from build123d import *

# Parameters (mm, degrees)
SKETCH1_R           = 49
BOSS_EXTRUDE1_DEPTH = 24.5
SKETCH2_R           = 24
BOSS_EXTRUDE2_DEPTH = 1.7
SKETCH3_R           = 18.5
BOSS_EXTRUDE3_DEPTH = 0.8
SKETCH4_R           = 35.5
BOSS_EXTRUDE4_DEPTH = 11
CIRPATTERN1_COUNT   = 8
CIRPATTERN2_COUNT   = 6
SKETCH20_R          = 1.5
CUT_EXTRUDE1_DEPTH  = 3.5
SKETCH21_R          = 2
BOSS_EXTRUDE5_DEPTH = 2.5
CIRPATTERN3_COUNT   = 3


with BuildPart() as part:
    # Sketch1 → Boss-Extrude1 (new body)
    with BuildSketch(Plane(origin=(0, 0, 0), x_dir=(1, 0, 0), z_dir=(0, 1, 0))):
        Circle(SKETCH1_R)
    extrude(amount=BOSS_EXTRUDE1_DEPTH)

    # Sketch2 → Boss-Extrude2 (add)
    with BuildSketch(Plane(origin=(0, 24.5, 0), x_dir=(1, 0, 0), z_dir=(0, 1, 0))):
        Circle(SKETCH2_R)
    extrude(amount=BOSS_EXTRUDE2_DEPTH)

    # Sketch3 → Boss-Extrude3 (add)
    with BuildSketch(Plane(origin=(0, 26.2, 0), x_dir=(1, 0, 0), z_dir=(0, 1, 0))):
        Circle(SKETCH3_R)
    extrude(amount=BOSS_EXTRUDE3_DEPTH)

    # Sketch4 → Boss-Extrude4 (add)
    with BuildSketch(Plane.XZ):
        Circle(SKETCH4_R)
    extrude(amount=BOSS_EXTRUDE4_DEPTH)

    # Sketch13 → 3.0mm Dowel Hole1 (revolve, cut)
    with BuildSketch(Plane(origin=(-39.264880132, 0, 16.264045876), x_dir=(0, 0, -1), z_dir=(1, 0, 0))):
        Polygon((0, 0), (0, 3.901290929), (1.5, 3), (1.5, 0), align=None)
    f_3_0mm_dowel_hole1 = revolve(axis=Axis((-39.264880132, -6.35, 16.264045876), (0, 1, 0)), mode=Mode.SUBTRACT)

    # CirPattern1: 3.0mm Dowel Hole1 ×8 about axis
    cirpattern1_axis = Axis((0, 0, 0), (0, 1, 0))
    for i in range(1, CIRPATTERN1_COUNT):
        add(f_3_0mm_dowel_hole1.rotate(cirpattern1_axis, i * 360 / CIRPATTERN1_COUNT), mode=Mode.SUBTRACT)

    # Sketch15 → 4.0mm Dowel Hole1 (revolve, cut)
    with BuildSketch(Plane(origin=(-15, 27, 0), x_dir=(0, 0, 1), z_dir=(1, 0, 0))):
        Polygon((0, 0), (0, 5.701721238), (2, 4.5), (2, 0), align=None)
    f_4_0mm_dowel_hole1 = revolve(axis=Axis((-15, 33.35, 0), (0, -1, 0)), mode=Mode.SUBTRACT)

    # CirPattern2: 4.0mm Dowel Hole1 ×6 about axis, 3 skipped
    cirpattern2_axis = Axis((0, -12.925, 0), (0, 1, 0))
    add([f_4_0mm_dowel_hole1.rotate(cirpattern2_axis, i * 360 / CIRPATTERN2_COUNT) for i in range(1, CIRPATTERN2_COUNT) if i not in (1, 3, 5)], mode=Mode.SUBTRACT)

    # Sketch20 → Cut-Extrude1 (cut)
    with BuildSketch(Plane(origin=(0, 24.5, 0), x_dir=(1, 0, 0), z_dir=(0, 1, 0))):
        with Locations((39.264880132, -16.264045876)):
            Circle(SKETCH20_R)
        with Locations((16.264045876, -39.264880132)):
            Circle(SKETCH20_R)
        with Locations((-16.264045876, -39.264880132)):
            Circle(SKETCH20_R)
        with Locations((-39.264880132, -16.264045876)):
            Circle(SKETCH20_R)
        with Locations((-39.264880132, 16.264045876)):
            Circle(SKETCH20_R)
        with Locations((-16.264045876, 39.264880132)):
            Circle(SKETCH20_R)
        with Locations((16.264045876, 39.264880132)):
            Circle(SKETCH20_R)
        with Locations((39.264880132, 16.264045876)):
            Circle(SKETCH20_R)
    extrude(amount=-CUT_EXTRUDE1_DEPTH, mode=Mode.SUBTRACT)

    # Sketch21 → Boss-Extrude5 (add)
    with BuildSketch(Plane(origin=(0, 27, 0), x_dir=(1, 0, 0), z_dir=(0, 1, 0))):
        with Locations((-7.125, 12.340862004)):
            Circle(SKETCH21_R)
    boss_extrude5 = extrude(amount=BOSS_EXTRUDE5_DEPTH)

    # CirPattern3: Boss-Extrude5 ×3 about axis
    cirpattern3_axis = Axis((0, 0, 0), (0, 1, 0))
    for i in range(1, CIRPATTERN3_COUNT):
        add(boss_extrude5.rotate(cirpattern3_axis, i * 360 / CIRPATTERN3_COUNT))


solid = part.part
Work out the finished part from the listing and answer in its coordinate system (mm). A direction names the side the tool comes from. Round coordinates to 2 decimals unless told otherwise and drop trailing zeros. Loops run counter-clockwise (first coordinate to the right, second up) from the corner with the lowest first, then second, coordinate; pieces in that order, holes last. Notation, with made-up numbers: (20.5, 66.5) - (40.5, 66.5) arc R21 cw to (40.5, 90.5) - close; hole circle Ø1 at (-32.75, 42.25). An arc over 180 degrees is marked (long way). One line per item, written item: value.
Q1. Find section A-A on x = 0. Give the vertices of the cut face in (y, z).
Check values:
outline: (-11, -35.5) - (0, -35.5) - (0, -49) - (24.5, -49) - (24.5, -24) - (26.2, -24) - (26.2, -18.5) - (27, -18.5) - (27, 18.5) - (26.2, 18.5) - (26.2, 24) - (24.5, 24) - (24.5, 49) - (0, 49) - (0, 35.5) - (-11, 35.5) - close
Q2. The mould has two halves that part along X. Classify faces 4 (the conical face through (-16.321, 3.745, -39.011)), 5 (the cylindrical face through (-7.696, -5.423, -34.656)), 6 (the flat face through (21, 24.5, -12)): +X half, -X half, draft (parallel to the pull), parting line (faces both ways), or undercut.
Check values:
face 4: undercut
face 5: parting line
face 6: draft
Q3. Find section D-D on z = 43. Give the vertices of the cut face in (x, y).
Check values:
outline: (-23.49, 0) - (23.49, 0) - (23.49, 24.5) - (-23.49, 24.5) - close
Q4. Each of these flat-tipped pins is pushed along its axis until it touches: pin 1 Ø1.5 at (x, z) = (-16, 40) entering from +Y; pin 2 Ø1.5 at (x, z) = (16.5, -39.5) entering from +Y; pin 3 Ø1.8 at (x, z) = (39.26, 16.26) entering from -Y. Where does it stop, or does it pass through?
Check values:
pin 1: y = 24.5
pin 2: y = 21
pin 3: y = 3.36
Q5. Straight lines are drawn through the part: probe 1 along Y at (x, z) = (25.5, 9); probe 2 along X at (y, z) = (23, 0); probe 3 along Y at (x, z) = (11, 42). For each, find the intervals that lie inside material, in ascending order.
Check values:
probe 1: -11 to 24.5
probe 2: -49 to -17, -13 to 49
probe 3: 0 to 24.5
Q6. Find section C-C on x = -32. Give the vertices of the cut face in (y, z), and give its area (3 significant figures).
Check values:
outline: (-11, -15.37) - (0, -15.37) - (0, -37.11) - (24.5, -37.11) - (24.5, 37.11) - (0, 37.11) - (0, 15.37) - (-11, 15.37) - close
area: 2,160 mm2
Q7. For faces 1 (the cylindrical face through (-8.71, 28.23, -11.12)), 2 (the flat face through (-7, 29.5, 12)), 3 (the cylindrical face through (16.59, 1.48, 37.8)), determine the directions among +Z, -Z, +X, -X, +Y, -Y from which every point of the face is accessible in a straight line to the end or side of a thin tool.
Check values:
face 1: +Y
face 2: +Z, -Z, +X, -X, +Y
face 3: -Y
Q8. Find section B-B on y = 19. Give the vertices of the cut face in (x, z).
Check values:
outline: circle Ø98 at (0, 0)
